Job drawing, mm, ordinate dimensions from the low corner. One solid piece. A direction names the side the tool comes from. Give positions to 0.01 mm unless a question says otherwise; leave off trailing zeros. Write each loop counter-clockwise with the first axis right and the second up, starting at its lowest first coordinate (ties: lowest second). Pieces come first, ordered by that corner, then holes. Notation, with made-up numbers: M -35.75,75 L 7.25,75 A10 cw 7.25,88 Z; hole C 44.25,-7 d8. An arc over 180 degrees is marked long. Answer as CSV lines item,"result". Start each with the question number.
Item 1: Band-saw the part on D-D, the plane x = 40. List the corners of the cut face in (y, z), then the cut area to 3 significant figures.
Item 2: Two-plate mould, pull along Y, no slides. Class the marked faces 4 and 5: +Y half, -Y half, draft (parallel to the pull), parting line (faces both ways), or undercut.
Item 3: Band-saw the part on A-A, the plane z = 8.75. List the corners of the cut face in (x, y), then the cut area to 3 significant figures.
Item 4: Band-saw the part on C-C, the plane x = 8. List the corners of the cut face in (y, z).
Item 5: 3-axis set-ups, long thin cutter, end or side, ignore diameter. For the marked faces 1, 2 and 3: which of +Z, -Z, +X, -X, +Y, -Y reach the whole face in a straight line?
Item 6: Wall check: L1, parallel to X at y = 8.25, z = 1; L2, parallel to Y at x = 22.5, z = 9; L3, parallel to Y at x = 23.5, z = 1.75. Give the ranges that are in metal, low to high. Write a range as from..to.
Item 7: Pin check, flat tips, straight feed: pin 1 (1.5 mm diameter, centred on x = 45.5, z = 12, fed in from -Y); pin 2 (8 mm diameter, centred on x = 33.5, z = 4, fed in from +Y); pin 3 (8 mm diameter, centred on x = 48.5, z = 5.5, fed in from +Y). Stop position of each tip, or through.
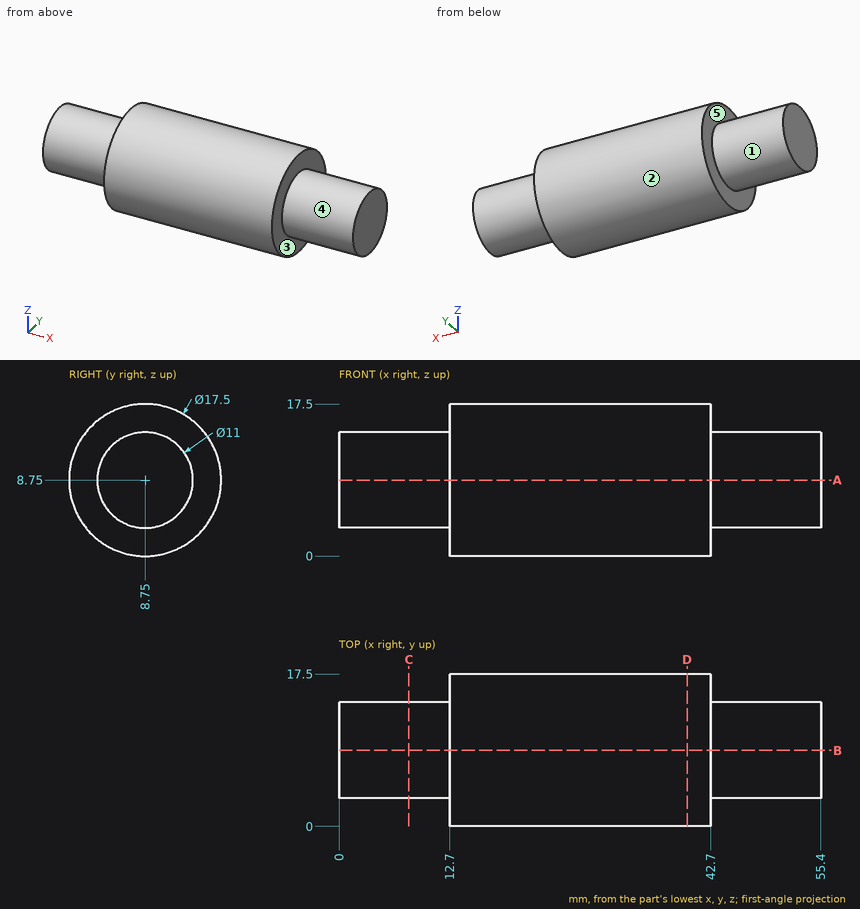
Output:
1,outline,"C 8.75,8.75 d17.5"
1,area,"241 mm²"
2,face 4,"parting line"
2,face 5,"draft"
3,outline,"M 0,3.25 L 12.7,3.25 L 12.7,0 L 42.7,0 L 42.7,3.25 L 55.4,3.25 L 55.4,14.25 L 42.7,14.25 L 42.7,17.5 L 12.7,17.5 L 12.7,14.25 L 0,14.25 Z"
3,area,"804 mm²"
4,outline,"C 8.75,8.75 d11"
5,face 1,"-X"
5,face 2,"+X, -X"
5,face 3,"+X"
6,L1,"12.7..42.7"
6,L2,"0..17.5"
6,L3,"3.5..14"
7,pin 1,"y = 3.85"
7,pin 2,"y = 17.47"
7,pin 3,"y = 14.25"
